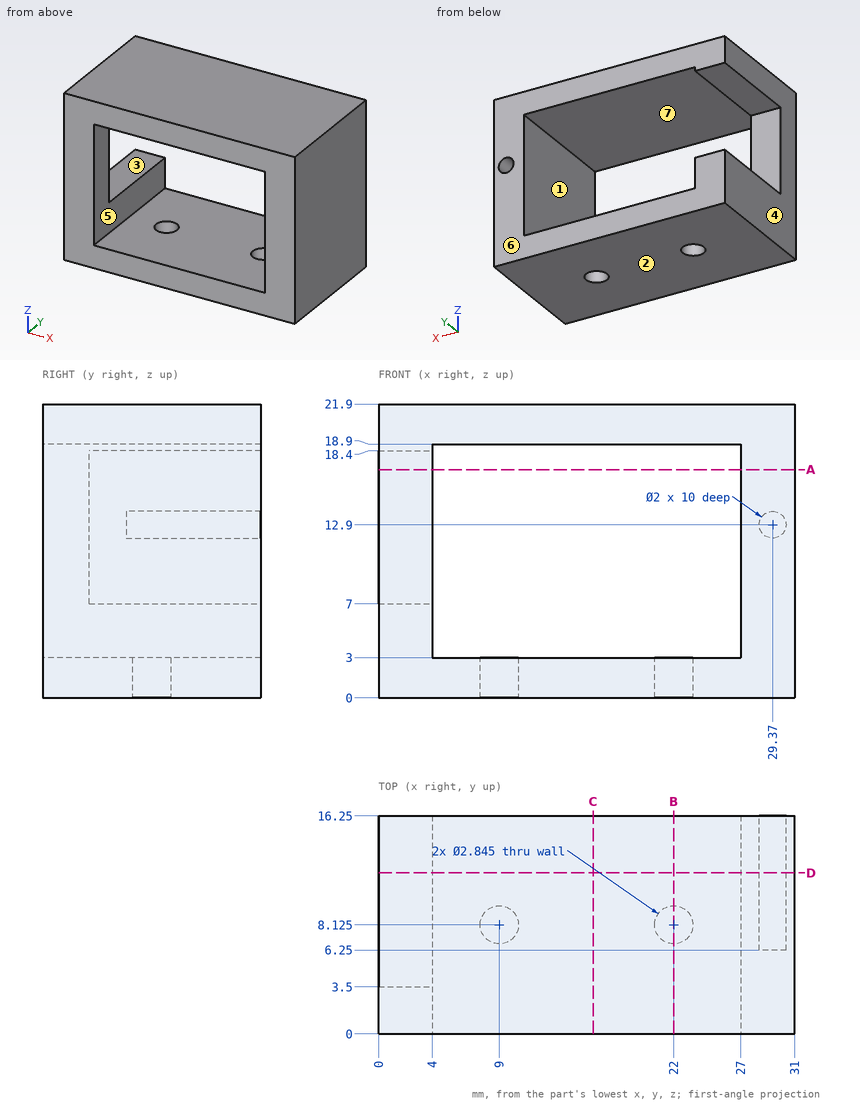
Drawing for the job (mm, zero at the part's lowest x, y, z). A direction names the side the tool comes from. Give positions to 0.01 mm unless a question says otherwise; leave off trailing zeros. Order: outer loops, then holes, each group sorted by start corner. A loop starts at its lowest first (then second) coordinate and runs counter-clockwise, first axis right, second up. Notation, with made-up numbers: M 61,66.5 L 90,66.5 A10 ccw 90,76.5 Z; hole C -19.75,81.5 d4. An arc over 180 degrees is marked long. Use a Markdown table: item, result. Add a question column.
(1) Probe line 1 along X through (y, z) = (1.5, 16.5); line 2 along Z through (x, y) = (7, 15.75); line 3 along Y through (x, z) = (9, 1.55). List the from-to ranges inside material, lowest first. Write a range as [from, to].
(2) 3-axis set-ups, long thin cutter, end or side, ignore diameter. For the marked faces 1, 2 and 3: which of +Z, -Z, +X, -X, +Y, -Y reach the whole face in a straight line?
(3) Mould opens along X. For the marked faces 4, 5, 6 and 7 say: +X half, -X half, draft (parallel to the pull), parting line (faces both ways), or undercut.
(4) Drop flat-ended pins along their axis: P1, Ø2.5, axis at x = 22, y = 8.125, coming from the -Z side; P2, Ø1.2, axis at x = 2.5, z = 11.5, coming from the +Y side; P3, Ø5, axis at y = 8.5, z = 13, coming from the -X side. Give the stop position or say it passes through.
(5) Saw through at A-A, the plane z = 17. Give the cut face in (x, y), and give its area (3 significant figures).
(6) Saw through at D-D, the plane y = 12. Give the cut face in (x, z).
(7) Saw through at B-B, the plane x = 22. Give the cut face in (y, z).
(8) Saw through at C-C, the plane x = 16. Give the cut face in (y, z), and give its area (3 significant figures).
Answer key:
| question | item | result |
|---|---|---|
| 1 | line 1 | [0, 4], [27, 31] |
| 1 | line 2 | [0, 3], [18.9, 21.9] |
| 1 | line 3 | [0, 6.7], [9.55, 16.25] |
| 2 | face 1 | +Y, -Y |
| 2 | face 2 | -Z, +X, -X, +Y, -Y |
| 2 | face 3 | -X, +Y |
| 3 | face 4 | -X half |
| 3 | face 5 | undercut |
| 3 | face 6 | draft |
| 3 | face 7 | undercut |
| 4 | P1 | z = 18.9 |
| 4 | P2 | y = 3.5 |
| 4 | P3 | x = 27 |
| 5 | outline | M 0,0 L 4,0 L 4,3.5 L 0,3.5 Z; M 27,0 L 31,0 L 31,16.25 L 27,16.25 Z |
| 5 | area | 79.0 mm^2 |
| 6 | outline | M 0,0 L 31,0 L 31,21.9 L 0,21.9 L 0,18.4 L 4,18.4 L 4,18.9 L 27,18.9 L 27,3 L 4,3 L 4,7 L 0,7 Z; hole C 29.37,12.9 d2 |
| 7 | outline | M 0,0 L 6.7,0 L 6.7,3 L 0,3 Z; M 0,18.9 L 16.25,18.9 L 16.25,21.9 L 0,21.9 Z; M 9.55,0 L 16.25,0 L 16.25,3 L 9.55,3 Z |
| 8 | outline | M 0,0 L 16.25,0 L 16.25,3 L 0,3 Z; M 0,18.9 L 16.25,18.9 L 16.25,21.9 L 0,21.9 Z |
| 8 | area | 97.5 mm^2 |
